from build123d import *

# Parameters (mm, degrees)
SKETCH1_W           = 116.1
SKETCH1_H           = 47.7
BOSS_EXTRUDE1_DEPTH = 3.9
SKETCH4_R           = 1.65
CUT_EXTRUDE3_DEPTH  = 4.9
SKETCH5_R           = 1.65
CUT_EXTRUDE4_DEPTH  = 4.9
SKETCH7_W           = 116.1
SKETCH7_H           = 3.9
BOSS_EXTRUDE2_DEPTH = 80
SKETCH8_R           = 2
CUT_EXTRUDE5_DEPTH  = 4.9
SKETCH9_R           = 1
CUT_EXTRUDE6_DEPTH  = 4.9


with BuildPart() as part:
    # Sketch1 → Boss-Extrude1 (new body)
    with BuildSketch(Plane(origin=(0, 0, 0), x_dir=(1, 0, 0), z_dir=(0, 1, 0))):
        with Locations((58.05, 23.85)):
            Rectangle(SKETCH1_W, SKETCH1_H)
    extrude(amount=BOSS_EXTRUDE1_DEPTH)

    # Sketch4 → Cut-Extrude3 (cut, through all)
    with BuildSketch(Plane(origin=(0, 3.9, 0), x_dir=(1, 0, 0), z_dir=(0, 1, 0))):
        with Locations((3, 42.7)):
            Circle(SKETCH4_R)
    cut_extrude3 = extrude(amount=-CUT_EXTRUDE3_DEPTH, mode=Mode.SUBTRACT)

    # Sketch5 → Cut-Extrude4 (cut, through all)
    with BuildSketch(Plane(origin=(0, 3.9, 0), x_dir=(1, 0, 0), z_dir=(0, 1, 0))):
        with Locations((3, 5)):
            Circle(SKETCH5_R)
    cut_extrude4 = extrude(amount=-CUT_EXTRUDE4_DEPTH, mode=Mode.SUBTRACT)

    # Mirror1: Cut-Extrude3, Cut-Extrude4 across plane
    add(cut_extrude3.mirror(Plane.ZY.offset(-58.05)), mode=Mode.SUBTRACT)
    add(cut_extrude4.mirror(Plane.ZY.offset(-58.05)), mode=Mode.SUBTRACT)

    # Sketch7 → Boss-Extrude2 (add)
    with BuildSketch(Plane.XY):
        with Locations((58.05, 1.95)):
            Rectangle(SKETCH7_W, SKETCH7_H)
    extrude(amount=BOSS_EXTRUDE2_DEPTH)

    # Sketch8 → Cut-Extrude5 (cut, through all)
    with BuildSketch(Plane(origin=(0, 3.9, 0), x_dir=(1, 0, 0), z_dir=(0, 1, 0))):
        with Locations((54.2, -54.7)):
            Circle(SKETCH8_R)
        with Locations((54.2, 12.5)):
            Circle(SKETCH8_R)
    extrude(amount=-CUT_EXTRUDE5_DEPTH, mode=Mode.SUBTRACT)

    # Sketch9 → Cut-Extrude6 (cut, through all)
    with BuildSketch(Plane(origin=(0, 3.9, 0), x_dir=(1, 0, 0), z_dir=(0, 1, 0))):
        with Locations((36.5, -65.5)):
            Circle(SKETCH9_R)
        with Locations((36.5, -55.5)):
            Circle(SKETCH9_R)
    extrude(amount=-CUT_EXTRUDE6_DEPTH, mode=Mode.SUBTRACT)


solid = part.part
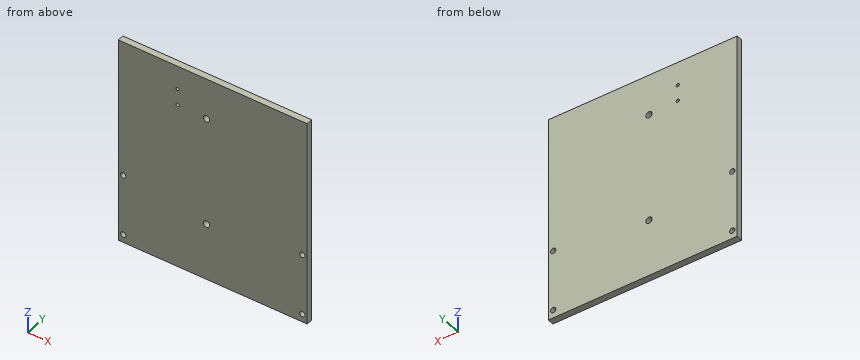
Could you check a few things on this model? Use its own coordinates, in mm. Coordinates: 2 decimals unless noted, no trailing zeros. Order: outer loops, then holes, each group sorted by start corner. A loop starts at its lowest first (then second) coordinate and runs counter-clockwise, first axis right, second up.
Q1. Will this pin go through, and if not, where does the flat tip stop? pin 1 (2 mm diameter, centred on x = 3, z = -5, fed in from +Y).
Q2. Suppose I cut it at A-A on x = 3. Please give me the cut outline in (y, z), and give its area (3 significant figures).
Q3. Suppose I cut it at C-C on z = -42.7. Please give me the cut outline in (x, y), and give its area (3 significant figures).
Q4. Suppose I cut it at B-B on z = -12.5. Please give me the cut outline in (x, y), and give its area (3 significant figures).
Q5. Please list where these lines run through material, in increasing order: L1, parallel to Z at x = 54.2, y = 1.7; L2, parallel to Z at x = 36.5, y = 2.9; L3, parallel to X at y = 2.4, z = 65.5.
Answer:
1. pin 1: passes through
2. outline: (0, -47.7) - (3.9, -47.7) - (3.9, -44.35) - (0, -44.35) - close; (0, -41.05) - (3.9, -41.05) - (3.9, -6.65) - (0, -6.65) - close; (0, -3.35) - (3.9, -3.35) - (3.9, 80) - (0, 80) - close
2. area: 472 mm2
3. outline: (0, 0) - (1.35, 0) - (1.35, 3.9) - (0, 3.9) - close; (4.65, 0) - (111.45, 0) - (111.45, 3.9) - (4.65, 3.9) - close; (114.75, 0) - (116.1, 0) - (116.1, 3.9) - (114.75, 3.9) - close
3. area: 427 mm2
4. outline: (0, 0) - (52.2, 0) - (52.2, 3.9) - (0, 3.9) - close; (56.2, 0) - (116.1, 0) - (116.1, 3.9) - (56.2, 3.9) - close
4. area: 437 mm2
5. L1: z = -47.7 to -14.5, -10.5 to 52.7, 56.7 to 80
5. L2: z = -47.7 to 54.5, 56.5 to 64.5, 66.5 to 80
5. L3: x = 0 to 35.5, 37.5 to 116.1
